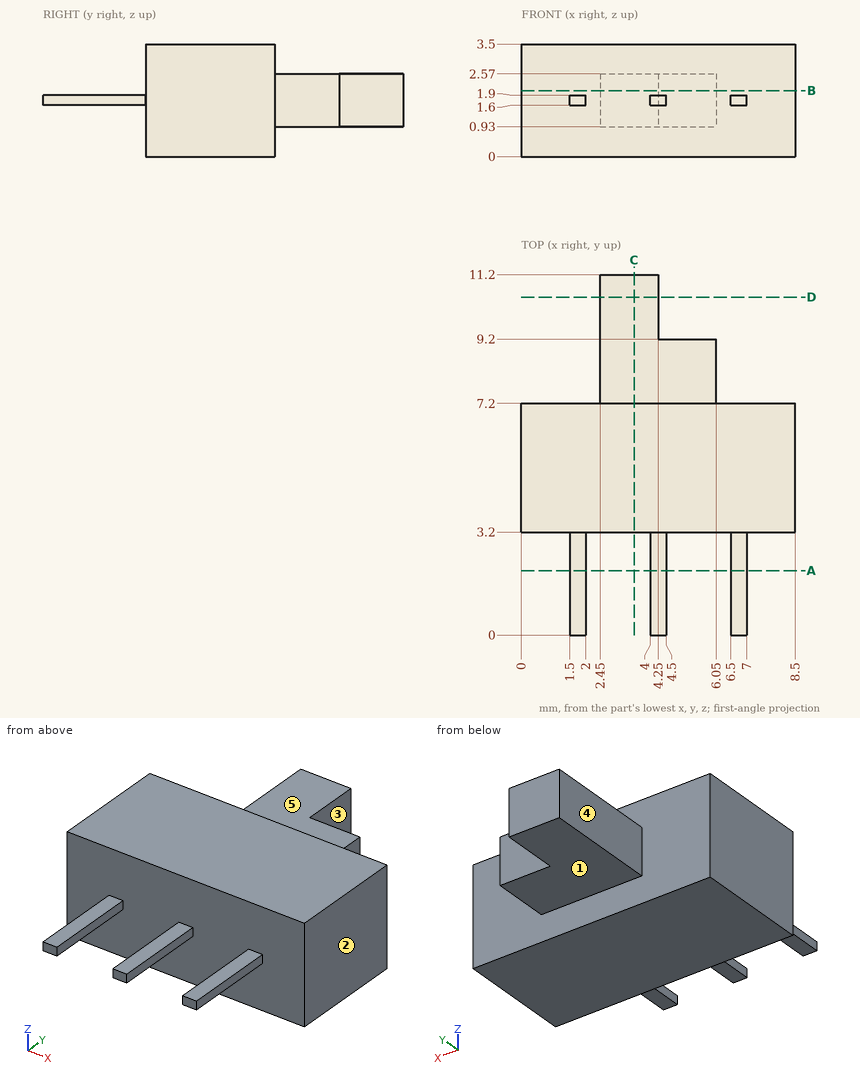
Here's the drawing with two shaded views (mm, measured from the low corner). I have some questions. A direction names the side the tool comes from. Give positions to 0.01 mm unless a question says otherwise; leave off trailing zeros. Write each loop counter-clockwise with the first axis right and the second up, starting at its lowest first coordinate (ties: lowest second). Pieces come first, ordered by that corner, then holes. Notation, with made-up numbers: (-14, 21) - (-9, 21) arc R26 ccw to (-9, 42) - close; hole circle Ø10 at (-14.5, 80.5). An arc over 180 degrees is marked (long way). One line per item, written item: value. Start each with the question number.
Item 1: Imagine slicing it at D-D, the plane y = 10.5. List the corners of the cut face in (x, z) for me, and give its area (3 significant figures).
Item 2: Imagine slicing it at B-B, the plane z = 2.05. List the corners of the cut face in (x, y) for me, and give its area (3 significant figures).
Item 3: Imagine slicing it at A-A, the plane y = 2. List the corners of the cut face in (x, z) for me, and give its area (3 significant figures).
Item 4: Which directions (+Z, -Z, +X, -X, +Y, -Y) give clear straight access to the entire face, cutting with the end or side of a thin tool? Please do the marked faces 1, 2, 3, 4 and 5.
Item 5: Imagine slicing it at C-C, the plane x = 3.5. List the corners of the cut face in (y, z) for me, and give its area (3 significant figures).
Item 6: Please list where these lines run through material, in increasing order: line 1 (X direction, y = 3, z = 1.85); line 2 (Y direction, x = 8, z = 2.95); line 3 (Z direction, x = 5.75, y = 8.25). Write a range as from..to.
Item 7: I'm going to push flat-ended pins straight in: pin 1 (1.1 mm diameter, centred on x = 4, y = 8.5, fed in from -Z); pin 2 (1.5 mm diameter, centred on x = 2, z = 0.5, fed in from -Y); pin 3 (1.1 mm diameter, centred on x = 4.5, y = 8.5, fed in from +Z). Where does each tip first touch, or does it pass through?
Geometry says:
1. outline: (2.45, 0.93) - (4.25, 0.93) - (4.25, 2.57) - (2.45, 2.57) - close
1. area: 2.95 mm^2
2. outline: (0, 3.2) - (8.5, 3.2) - (8.5, 7.2) - (6.05, 7.2) - (6.05, 9.2) - (4.25, 9.2) - (4.25, 11.2) - (2.45, 11.2) - (2.45, 7.2) - (0, 7.2) - close
2. area: 44.8 mm^2
3. outline: (1.5, 1.6) - (2, 1.6) - (2, 1.9) - (1.5, 1.9) - close; (4, 1.6) - (4.5, 1.6) - (4.5, 1.9) - (4, 1.9) - close; (6.5, 1.6) - (7, 1.6) - (7, 1.9) - (6.5, 1.9) - close
3. area: 0.450 mm^2
4. face 1: -Z, +X, -X, +Y
4. face 2: +Z, -Z, +X, +Y, -Y
4. face 3: +Z, -Z, +X, +Y
4. face 4: +Z, -Z, -X, +Y
4. face 5: +Z, +X, -X, +Y
5. outline: (3.2, 0) - (7.2, 0) - (7.2, 0.93) - (11.2, 0.93) - (11.2, 2.57) - (7.2, 2.57) - (7.2, 3.5) - (3.2, 3.5) - close
5. area: 20.6 mm^2
6. line 1: 1.5..2, 4..4.5, 6.5..7
6. line 2: 3.2..7.2
6. line 3: 0.93..2.57
7. pin 1: z = 0.93
7. pin 2: y = 3.2
7. pin 3: z = 2.57
